```python
from build123d import *

# Parameters (mm, degrees)
SKETCH1_R           = 37.5
SKETCH1_R_2         = 32.5
SKETCH1_W           = 5
SKETCH1_H           = 5
SKETCH1_R_3         = 0.5
BOSS_EXTRUDE1_DEPTH = 1
SKETCH2_R           = 37.5
SKETCH2_R_2         = 35.5
BOSS_EXTRUDE2_DEPTH = 2


with BuildPart() as part:
    # Sketch1 → Boss-Extrude1 (new body)
    # profile 1 of 6: a face of its own
    with BuildSketch(Plane(origin=(0, 0, 0), x_dir=(1, 0, 0), z_dir=(0, 1, 0))):
        with Locations(Location((0, 0, 0), (0, 0, 270))):
            Circle(SKETCH1_R)
        Circle(SKETCH1_R_2, mode=Mode.SUBTRACT)
    # profile 2 of 6: a face of its own
    with BuildSketch(Plane(origin=(0, 0, 0), x_dir=(1, 0, 0), z_dir=(0, 1, 0))):
        with BuildLine():
            ThreePointArc((2.5, 32.403703492), (0, 32.5), (-2.5, 32.403703492))
            Line((-2.5, 32.403703492), (-2.5, 2.5))
            Line((-2.5, 2.5), (2.5, 2.5))
            Line((2.5, 2.5), (2.5, 32.403703492))
        make_face()
    # profile 3 of 6: a face of its own
    with BuildSketch(Plane(origin=(0, 0, 0), x_dir=(1, 0, 0), z_dir=(0, 1, 0))):
        with BuildLine():
            Line((2.5, -2.5), (-2.5, -2.5))
            Line((-2.5, -2.5), (-2.5, -32.403703492))
            ThreePointArc((-2.5, -32.403703492), (0, -32.5), (2.5, -32.403703492))
            Line((2.5, -32.403703492), (2.5, -2.5))
        make_face()
    # profile 4 of 6: a face of its own
    with BuildSketch(Plane(origin=(0, 0, 0), x_dir=(1, 0, 0), z_dir=(0, 1, 0))):
        with BuildLine():
            Line((-2.5, -2.5), (-2.5, 2.5))
            Line((-2.5, 2.5), (-32.403703492, 2.5))
            ThreePointArc((-32.403703492, 2.5), (-32.5, 0), (-32.403703492, -2.5))
            Line((-32.403703492, -2.5), (-2.5, -2.5))
        make_face()
    # profile 5 of 6: a face of its own
    with BuildSketch(Plane(origin=(0, 0, 0), x_dir=(1, 0, 0), z_dir=(0, 1, 0))):
        with BuildLine():
            Line((32.403703492, 2.5), (2.5, 2.5))
            Line((2.5, 2.5), (2.5, -2.5))
            Line((2.5, -2.5), (32.403703492, -2.5))
            ThreePointArc((32.403703492, -2.5), (32.47591695, -1.250926958), (32.5, 0))
            ThreePointArc((32.5, 0), (32.47591695, 1.250926958), (32.403703492, 2.5))
        make_face()
    # profile 6 of 6: a face of its own
    with BuildSketch(Plane(origin=(0, 0, 0), x_dir=(1, 0, 0), z_dir=(0, 1, 0))):
        Rectangle(SKETCH1_W, SKETCH1_H)
        with Locations(Location((0, 0, 0), (0, 0, 270))):
            Circle(SKETCH1_R_3, mode=Mode.SUBTRACT)
    extrude(amount=BOSS_EXTRUDE1_DEPTH)

    # Sketch2 → Boss-Extrude2 (add)
    with BuildSketch(Plane(origin=(0, 1, 0), x_dir=(1, 0, 0), z_dir=(0, 1, 0))):
        with Locations(Location((0, 0, 0), (0, 0, 270))):
            Circle(SKETCH2_R)
        with Locations(Location((0, 0, 0), (0, 0, 270))):
            Circle(SKETCH2_R_2, mode=Mode.SUBTRACT)
    extrude(amount=BOSS_EXTRUDE2_DEPTH)


solid = part.part
```
Could you check a few things on this model? Use its own coordinates, in mm. A direction names the side the tool comes from. Round coordinates to 2 decimals unless told otherwise and drop trailing zeros. Loops run counter-clockwise (first coordinate to the right, second up) from the corner with the lowest first, then second, coordinate; pieces in that order, holes last. Notation, with made-up numbers: (-27.5, 58) - (-5.5, 58) arc R10 ccw to (-5.5, 67) - close; hole circle Ø3 at (12, 53.25). An arc over 180 degrees is marked (long way). Answer in a Markdown table with one row per item. Add a question column.
(1) If we mould it in two halves opening along X, with no side actions, what happens to faces 3 (the face through (-1, 0, -1)), 4 (the face through (-31.495, 1.986, 16.381)), 5 (the face through (-22.818, 1.479, -29.759)), 6 (the face through (0, 1, -3))? For each: pulls with the +X half, pulls with the -X half, needs draft (parallel to the pull), parting line crosses it, or undercut.
(2) If we section it at A-A (z = 15): Please give me the cut outline in (x, y), plus the area to 3 significant figures.
(3) If we section it at B-B (x = -16): Please give me the cut outline in (y, z), plus the area to 3 significant figures.
(4) For faces 1 (the face through (-33, 3, 14)), 2 (the face through (-22.75, 0.49, -23.21)), which set-ups out of +Z, -Z, +X, -X, +Y, -Y let a thin tool reach every point of the face, with its end or its side?
(5) If we section it at C-C (y = 2.3): Please give me the cut outline in (x, z), plus the area to 3 significant figures.
(6) I need wall thicknesses on line 1 along X through (y, z) = (0.5, 0); line 2 along Z through (x, y) = (7.5, 0.1); line 3 along X through (y, z) = (0.8, -18). Which ranges of each line are inside material? Lowest first, please.
(7) I'm going to push flat-ended pins straight in: pin 1 (0.5 mm diameter, centred on x = -23, y = 0.5, fed in from -Z); pin 2 (1 mm diameter, centred on y = 2.5, z = -21, fed in from -X); pin 3 (0.5 mm diameter, centred on y = 0.5, z = -10.5, fed in from +X). Where does each tip first touch, or does it pass through?
Model answer:
| question | item | result |
|---|---|---|
| 1 | face 3 | needs draft |
| 1 | face 4 | undercut |
| 1 | face 5 | parting line crosses it |
| 1 | face 6 | undercut |
| 2 | outline | (-34.37, 0) - (-28.83, 0) - (-28.83, 1) - (-32.18, 1) - (-32.18, 3) - (-34.37, 3) - close; (-2.5, 0) - (2.5, 0) - (2.5, 1) - (-2.5, 1) - close; (28.83, 0) - (34.37, 0) - (34.37, 3) - (32.18, 3) - (32.18, 1) - (28.83, 1) - close |
| 2 | area | 24.9 mm² |
| 3 | outline | (0, -33.92) - (3, -33.92) - (3, -31.69) - (1, -31.69) - (1, -28.29) - (0, -28.29) - close; (0, -2.5) - (1, -2.5) - (1, 2.5) - (0, 2.5) - close; (0, 28.29) - (1, 28.29) - (1, 31.69) - (3, 31.69) - (3, 33.92) - (0, 33.92) - close |
| 3 | area | 25.2 mm² |
| 4 | face 1 | +Z, -Z, +X, -X, +Y |
| 4 | face 2 | +Y, -Y |
| 5 | outline | circle Ø75 at (0, 0); hole circle Ø71 at (0, 0) |
| 5 | area | 459 mm² |
| 6 | line 1 | x = -37.5 to -0.5, 0.5 to 37.5 |
| 6 | line 2 | z = -36.74 to -31.62, -2.5 to 2.5, 31.62 to 36.74 |
| 6 | line 3 | x = -32.9 to -27.06, -2.5 to 2.5, 27.06 to 32.9 |
| 7 | pin 1 | stops at z = -29.81 |
| 7 | pin 2 | stops at x = -31.4 |
| 7 | pin 3 | stops at x = 36.07 |
